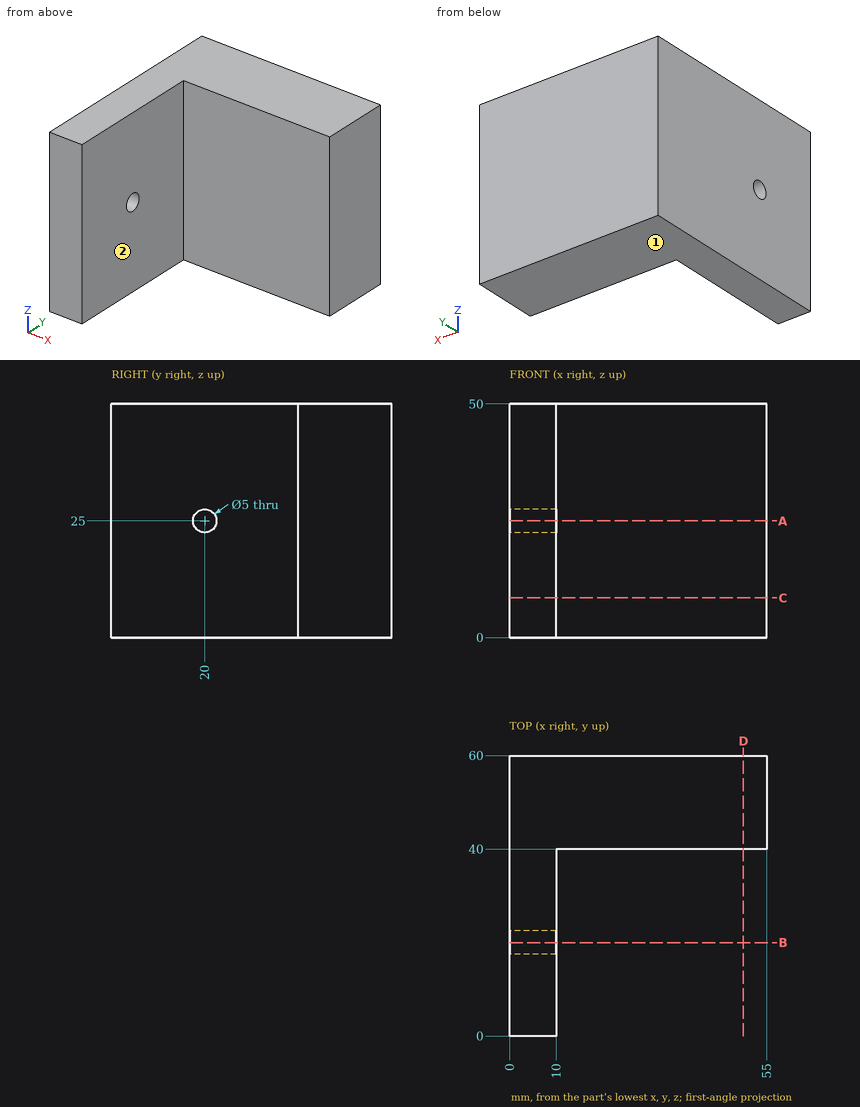
Check sheet for the drawn part. Datum: minimum x, y, z corner. Units: mm. A direction names the side the tool comes from. Round coordinates to 2 decimals unless told otherwise and drop trailing zeros. Order: outer loops, then holes, each group sorted by start corner. A loop starts at its lowest first (then second) coordinate and runs counter-clockwise, first axis right, second up. Notation, with made-up numbers: (50, 13.25) -> (89, 13.25) arc R22 cw to (89, 40.25) -> close; hole circle Ø1 at (59, -3.5). An arc over 180 degrees is marked (long way). Return JSON: item names as keys, results as strings. Group by question number.
Q1. Section check A-A, the plane z = 25. Record the boundary of the cut face in (x, y), plus the area to 3 significant figures.
Q2. Tool access check on the marked faces 1 and 2. Record the directions out of +Z, -Z, +X, -X, +Y, -Y that give a thin tool (end or side, any length) a straight path to the whole face; none if there is none.
Q3. Material ranges on probe 1 along Y at (x, z) = (3.25, 25); probe 2 along Y at (x, z) = (20, 24.5); probe 3 along X at (y, z) = (5.5, 2.5), recorded low to high. Write a range as from..to.
Q4. Gauge pin test, flat ends, axial feed: pin 1 (2 mm diameter, centred on x = 46, z = 34.5, fed in from -Y); pin 2 (1 mm diameter, centred on y = 11.5, z = 22, fed in from -X); pin 3 (12 mm diameter, centred on y = 26, z = 20.5, fed in from +X). Record the tip position at first contact, or that the pin passes through.
Q5. Section check C-C, the plane z = 8.5. Record the boundary of the cut face in (x, y), plus the area to 3 significant figures.
Q6. Section check D-D, the plane x = 50. Record the boundary of the cut face in (y, z), plus the area to 3 significant figures.
Q7. Section check B-B, the plane y = 20. Record the boundary of the cut face in (x, z).
Numbers:
{
 "1": {"outline": "(0, 0) -> (10, 0) -> (10, 17.5) -> (0, 17.5) -> close; (0, 22.5) -> (10, 22.5) -> (10, 40) -> (55, 40) -> (55, 60) -> (0, 60) -> close", "area": "1,450 mm^2"},
 "2": {"face 1": "-Z, +X, -X, +Y, -Y", "face 2": "+Z, -Z, +X, -Y"},
 "3": {"probe 1": "0..17.5, 22.5..60", "probe 2": "40..60", "probe 3": "0..10"},
 "4": {"pin 1": "y = 40", "pin 2": "x = 0", "pin 3": "x = 10"},
 "5": {"outline": "(0, 0) -> (10, 0) -> (10, 40) -> (55, 40) -> (55, 60) -> (0, 60) -> close", "area": "1,500 mm^2"},
 "6": {"outline": "(40, 0) -> (60, 0) -> (60, 50) -> (40, 50) -> close", "area": "1,000 mm^2"},
 "7": {"outline": "(0, 0) -> (10, 0) -> (10, 22.5) -> (0, 22.5) -> close; (0, 27.5) -> (10, 27.5) -> (10, 50) -> (0, 50) -> close"}
}
